Check sheet for the drawn part. Datum: minimum x, y, z corner. Units: mm. A direction names the side the tool comes from. Give positions to 0.01 mm unless a question says otherwise; leave off trailing zeros. Order: outer loops, then holes, each group sorted by start corner. A loop starts at its lowest first (then second) coordinate and runs counter-clockwise, first axis right, second up.
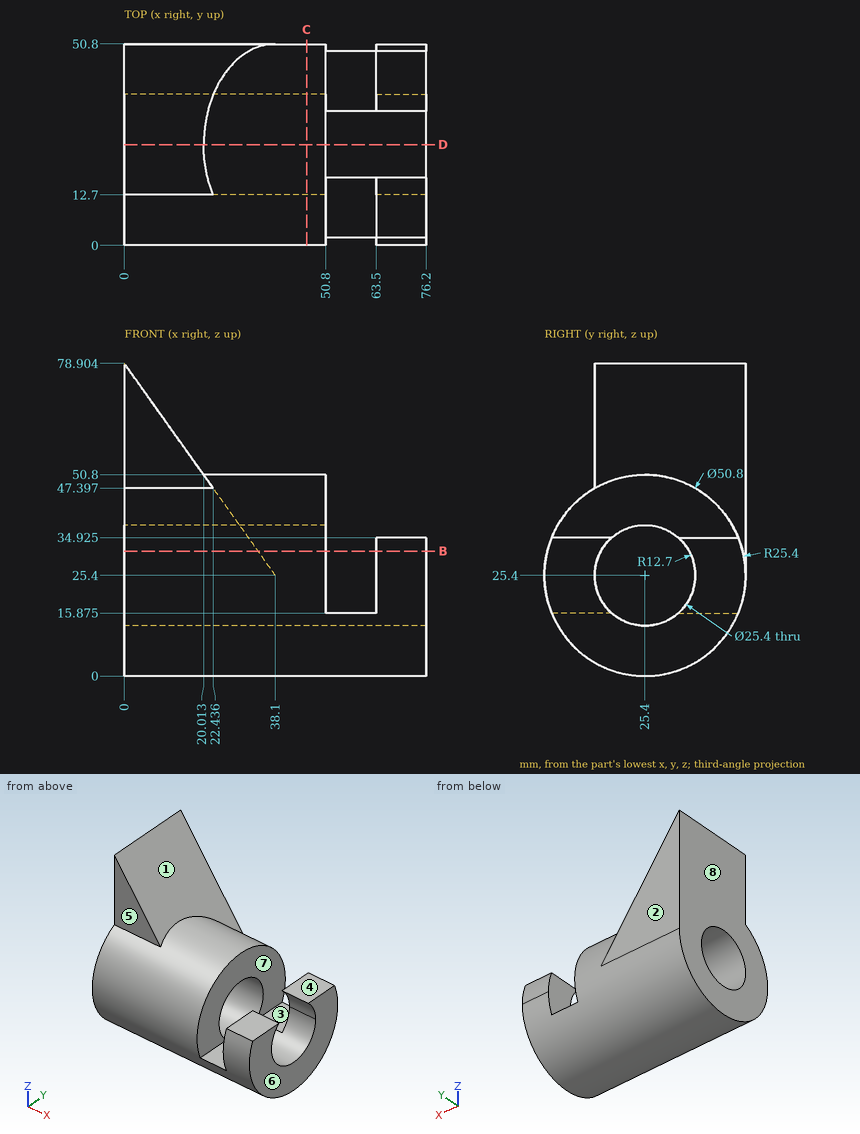
Item 1: Sectioned sample at B-B (z = 31.5). Enter the section's corners in (x, y), and give its area (3 significant figures).
Reported:
outline: (0, 0.74) - (50.8, 0.74) - (50.8, 14.26) - (0, 14.26) - close; (0, 36.54) - (50.8, 36.54) - (50.8, 50.06) - (33.76, 50.06) - (33.76, 50.8) - (0, 50.8) - close; (63.5, 0.74) - (76.2, 0.74) - (76.2, 14.26) - (63.5, 14.26) - close; (63.5, 36.54) - (76.2, 36.54) - (76.2, 50.06) - (63.5, 50.06) - close
area: 1,740 mm2
Item 2: Sectioned sample at C-C (x = 46). Enter the section's corners in (y, z), and give its area (3 significant figures).
Reported:
outline: circle Ø50.8 at (25.4, 25.4); hole circle Ø25.4 at (25.4, 25.4)
area: 1,520 mm2
Item 3: Draft check along X on the marked faces 1, 2 and 3. Enter one of: released by +X, released by -X, zero draft, split by the parting line, or undercut.
Reported:
face 1: released by +X
face 2: zero draft
face 3: undercut
Item 4: Set-up check for the marked faces 4, 5, 6, 7 and 8: record each of +Z, -Z, +X, -X, +Y, -Y from which the full face is reachable in a straight line by a thin tool's end or side.
Reported:
face 4: +Z, +X, +Y, -Y
face 5: +Z, +X, -X, -Y
face 6: +Z, -Z, +X, +Y, -Y
face 7: +Z, +Y, -Y
face 8: +Z, -Z, -X, +Y, -Y
Item 5: Gauge pin test, flat ends, axial feed: pin 1 (10 mm diameter, centred on x = 60, y = 6, fed in from +Z) (3 decimals); pin 2 (4 mm diameter, centred on x = 18.5, y = 25, fed in from +Z) (1 decimal); pin 3 (2 mm diameter, centred on x = 65, z = 23.5, fed in from -Y). Record the tip position at first contact, or that the pin passes through.
Reported:
pin 1: stops at z = 34.925
pin 2: stops at z = 55.7
pin 3: stops at y = 0.02
Item 6: Sectioned sample at D-D (y = 25.4). Enter the section's corners in (x, z) (1 decimal), and give its area (3 significant figures).
Reported:
outline: (0, 0) - (76.2, 0) - (76.2, 12.7) - (0, 12.7) - close; (0, 38.1) - (50.8, 38.1) - (50.8, 50.8) - (20, 50.8) - (0, 78.9) - close
area: 1,890 mm2
Item 7: Scan lines: L1, parallel to Y at x = 44.5, z = 25.4; L2, parallel to Z at x = 61, y = 25. Record each from-to range of solid material in increasing order.
Reported:
L1: y = 0 to 12.7, 38.1 to 50.8
L2: z = 0 to 12.71
